Work out the finished part from the listing and answer in its coordinate system (mm). Coordinates: 2 decimals unless noted, no trailing zeros. Write each loop counter-clockwise with the first axis right and the second up, starting at its lowest first coordinate (ties: lowest second). Pieces come first, ordered by that corner, then holes. Notation, with made-up numbers: (16, 61) - (37, 61) arc R25 cw to (37, 89) - close; hole circle Ø1 at (-4, 13). An arc over 180 degrees is marked (long way). One line per item, written item: value.
```python
from build123d import *

# Parameters (mm, degrees)
SKETCH1_R           = 16
BOSS_EXTRUDE1_DEPTH = 10.5
SKETCH2_R           = 16
BOSS_EXTRUDE2_DEPTH = 1.5
BOSS_EXTRUDE3_START = 10.5
SKETCH3_R           = 3.5
BOSS_EXTRUDE3_DEPTH = 10.5


with BuildPart() as part:
    # Sketch1 → Boss-Extrude1 (new body)
    with BuildSketch(Plane(origin=(0, 0, 0), x_dir=(1, 0, 0), z_dir=(0, 1, 0))):
        with Locations(Location((0, 0, 0), (0, 0, 90))):
            Circle(SKETCH1_R)
        with BuildLine():
            Line((-0.754325558, 14.480365774), (-0.751021188, 3.418474393))
            ThreePointArc((-0.751021188, 3.418474393), (-0.001045508, 3.499999844), (0.748978745, 3.418922468))
            Line((0.748978745, 3.418922468), (0.745674375, 14.480813849))
            ThreePointArc((0.745674375, 14.480813849), (12.5552021, 7.25375077), (12.917527395, -6.586917791))
            Line((12.917527395, -6.586917791), (3.335996261, -1.058833769))
            ThreePointArc((3.335996261, -1.058833769), (3.031611532, -1.749094486), (2.586384338, -2.358095854))
            Line((2.586384338, -2.358095854), (12.167915473, -7.886179876))
            ThreePointArc((12.167915473, -7.886179876), (0.004331389, -14.499999353), (-12.163201838, -7.893447983))
            Line((-12.163201838, -7.893447983), (-2.584975072, -2.359640624))
            ThreePointArc((-2.584975072, -2.359640624), (-3.030566024, -1.750905358), (-3.335363083, -1.060826614))
            Line((-3.335363083, -1.060826614), (-12.913589848, -6.594633973))
            ThreePointArc((-12.913589848, -6.594633973), (-12.559533489, 7.246248583), (-0.754325558, 14.480365774))
        make_face(mode=Mode.SUBTRACT)
    extrude(amount=BOSS_EXTRUDE1_DEPTH)

    # Sketch2 → Boss-Extrude2 (add)
    with BuildSketch(Plane(origin=(0, 10.5, 0), x_dir=(1, 0, 0), z_dir=(0, 1, 0))):
        with Locations(Location((0, 0, 0), (0, 0, 90))):
            Circle(SKETCH2_R)
    extrude(amount=BOSS_EXTRUDE2_DEPTH)

    # Sketch3 → Boss-Extrude3 (add)
    with BuildSketch(Plane.XZ.offset(-10.5).offset(BOSS_EXTRUDE3_START)):
        Circle(SKETCH3_R)
        with BuildLine():
            Line((-2.598076211, -1.5), (2.598076211, -1.5))
            ThreePointArc((2.598076211, -1.5), (0, 3), (-2.598076211, -1.5))
        make_face(mode=Mode.SUBTRACT)
    extrude(amount=-BOSS_EXTRUDE3_DEPTH)


solid = part.part
```
Item 1: Section A-A, the plane y = 5 is taken. Determine the outline of the cut face in (x, z).
Evaluation:
outline: circle Ø32 at (0, 0); hole (-12.91, 6.59) arc R14.5 ccw to (-0.75, -14.48) - (-0.75, -3.42) arc R3.5 cw to (-3.34, 1.06) - close; hole (-12.16, 7.89) - (-2.58, 2.36) arc R3.5 cw to (2.59, 2.36) - (12.17, 7.89) arc R14.5 ccw to start; hole (-2.6, -1.5) - (2.6, -1.5) arc R3 ccw (long way) to start; hole (0.75, -14.48) arc R14.5 ccw to (12.92, 6.59) - (3.34, 1.06) arc R3.5 cw to (0.75, -3.42) - close
Item 2: Determine the mould class of faces 1 (the face through (0, 12, 0)), 2 (the face through (15.62, 5.92, 3.47)), 3 (the face through (0, 5.2, 3.5)), 4 (the face through (0, 10.5, 0)) for opening direction X: +X half, -X half, draft (parallel to the pull), parting line (faces both ways), or undercut.
Evaluation:
face 1: draft
face 2: parting line
face 3: undercut
face 4: undercut
Item 3: Consider probe 1 along X at (y, z) = (6, 0); probe 2 along X at (y, z) = (8, -5.5); probe 3 along Z at (x, y) = (-6, 8.5). Determine where each line is inside the solid, lowest interval first.
Evaluation:
probe 1: x = -16 to -14.5, -3.5 to -3, 3 to 3.5, 14.5 to 16
probe 2: x = -15.02 to -13.42, -0.75 to 0.75, 13.42 to 15.02
probe 3: z = -14.83 to -13.2, 2.6 to 4.33, 13.2 to 14.83
Item 4: Section B-B, the plane x = 0 is taken. Determine the outline of the cut face in (y, z).
Evaluation:
outline: (0, -16) - (12, -16) - (12, 16) - (0, 16) - (0, 14.5) - (10.5, 14.5) - (10.5, 3.5) - (0, 3.5) - (0, 3) - (10.5, 3) - (10.5, -1.5) - (0, -1.5) - close
Item 5: Given pin 1 (1.3 mm diameter, centred on x = -0.5, z = 0, fed in from -Y); pin 2 (2 mm diameter, centred on x = 9, y = 6.5, fed in from +Z); pin 3 (6 mm diameter, centred on y = 2.5, z = -7, fed in from -X), each flat-ended and moving along its own axis, determine where each tip first touches the part or whether it passes through.
Evaluation:
pin 1: stops at y = 10.5
pin 2: stops at z = 13.86
pin 3: stops at x = -15.49
Item 6: Section C-C, the plane z = 0 is taken. Determine the outline of the cut face in (x, y), then the cut area to 3 significant figures.
Evaluation:
outline: (-16, 0) - (-14.5, 0) - (-14.5, 10.5) - (-3.5, 10.5) - (-3.5, 0) - (-3, 0) - (-3, 10.5) - (3, 10.5) - (3, 0) - (3.5, 0) - (3.5, 10.5) - (14.5, 10.5) - (14.5, 0) - (16, 0) - (16, 12) - (-16, 12) - close
area: 90.0 mm2
Item 7: Section D-D, the plane z = 7.5 is taken. Determine the outline of the cut face in (x, y), then the cut area to 3 significant figures.
Evaluation:
outline: (-14.13, 0) - (-11.48, 0) - (-11.48, 10.5) - (11.5, 10.5) - (11.5, 0) - (14.13, 0) - (14.13, 12) - (-14.13, 12) - close
area: 97.9 mm2
